Work out the finished part from the listing and answer in its coordinate system (mm). A direction names the side the tool comes from. Give positions to 0.01 mm unless a question says otherwise; leave off trailing zeros. Order: outer loops, then holes, each group sorted by start corner. A loop starts at its lowest first (then second) coordinate and runs counter-clockwise, first axis right, second up.
```python
from build123d import *

# Parameters (mm, degrees)
SKETCH_W      = 62.5
SKETCH_H      = 56.5
SKETCH_R      = 2.5
SKETCH_R_2    = 4
PAD_DEPTH     = 4
SKETCH001_R   = 19
SKETCH001_R_2 = 4
POCKET_DEPTH  = 1.5


with BuildPart() as part:
    # Sketch → Pad (new body)
    with BuildSketch(Plane.XY):
        Rectangle(SKETCH_W, SKETCH_H)
        with Locations((23.25, -23.25)):
            Circle(SKETCH_R, mode=Mode.SUBTRACT)
        with Locations((23.25, 23.25)):
            Circle(SKETCH_R, mode=Mode.SUBTRACT)
        with Locations((-23.25, 23.25)):
            Circle(SKETCH_R, mode=Mode.SUBTRACT)
        with Locations((-23.25, -23.25)):
            Circle(SKETCH_R, mode=Mode.SUBTRACT)
        Circle(SKETCH_R_2, mode=Mode.SUBTRACT)
    extrude(amount=PAD_DEPTH)

    # Sketch001 (on Face11 of Pad) → Pocket (cut)
    with BuildSketch(Plane.XY.offset(4)):
        Circle(SKETCH001_R)
        Circle(SKETCH001_R_2, mode=Mode.SUBTRACT)
    extrude(amount=-POCKET_DEPTH, mode=Mode.SUBTRACT)


solid = part.part
```
1. The part is cut by section A-A (y = 0). Write down the section's boundary in (x, z).
Findings below:
outline: (-31.25, 0) - (-4, 0) - (-4, 2.5) - (-19, 2.5) - (-19, 4) - (-31.25, 4) - close; (4, 0) - (31.25, 0) - (31.25, 4) - (19, 4) - (19, 2.5) - (4, 2.5) - close
2. Given P1, Ø6.5, axis at x = 0, y = 0, coming from the -Z side, flat-ended and moving along its own axis, determine where the tip first touches the part or whether it passes through.
Findings below:
P1: passes through
3. The part is cut by section D-D (x = 23.25). Write down the section's boundary in (y, z).
Findings below:
outline: (-28.25, 0) - (-25.75, 0) - (-25.75, 4) - (-28.25, 4) - close; (-20.75, 0) - (20.75, 0) - (20.75, 4) - (-20.75, 4) - close; (25.75, 0) - (28.25, 0) - (28.25, 4) - (25.75, 4) - close
4. The mould has two halves that part along Y. Classify faces 3 (the face through (0, 28.25, 2)), 4 (the face through (0, -28.25, 2)), 5 (the face through (8.767, -16.856, 3.26)), 6 (the face through (-0.4, 19.2, 4)): pulls with the +Y half, pulls with the -Y half, needs draft (parallel to the pull), parting line crosses it, or undercut.
Findings below:
face 3: pulls with the +Y half
face 4: pulls with the -Y half
face 5: undercut
face 6: needs draft
5. The part is cut by section B-B (x = 0). Write down the section's boundary in (y, z), then the cut area to 3 significant figures.
Findings below:
outline: (-28.25, 0) - (-4, 0) - (-4, 2.5) - (-19, 2.5) - (-19, 4) - (-28.25, 4) - close; (4, 0) - (28.25, 0) - (28.25, 4) - (19, 4) - (19, 2.5) - (4, 2.5) - close
area: 149 mm2
6. Which of the six approach directions +Z, -Z, +X, -X, +Y, -Y give full straight-line access (tool end or side, diameter ignored) to faces 1 (the face through (0, 7, 0)), 2 (the face through (-0.3, 4.5, 2.5))?
Findings below:
face 1: -Z, +X, -X, +Y, -Y
face 2: +Z
7. The part is cut by section C-C (z = 0.95). Write down the section's boundary in (x, y).
Findings below:
outline: (-31.25, -28.25) - (31.25, -28.25) - (31.25, 28.25) - (-31.25, 28.25) - close; hole circle Ø5 at (-23.25, -23.25); hole circle Ø5 at (-23.25, 23.25); hole circle Ø8 at (0, 0); hole circle Ø5 at (23.25, -23.25); hole circle Ø5 at (23.25, 23.25)
8. Straight lines are drawn through the part: probe 1 along Y at (x, z) = (23.25, 2.35); probe 2 along Y at (x, z) = (0, 3.1); probe 3 along Y at (x, z) = (0, 1.15). For each, find the intervals that lie inside material, in ascending order.
Findings below:
probe 1: y = -28.25 to -25.75, -20.75 to 20.75, 25.75 to 28.25
probe 2: y = -28.25 to -19, 19 to 28.25
probe 3: y = -28.25 to -4, 4 to 28.25
